from build123d import *

# Parameters (mm, degrees)
SKETCH1_W                 = 8.94
SKETCH1_H                 = 8.96
EXTRUDE1_DEPTH            = 2.85
M5X0_8_TAPPED_HOLE1_D     = 4.2
M5X0_8_TAPPED_HOLE1_DEPTH = 12.4
M5X0_8_TAPPED_HOLE1_TIP   = 1.2618073
CHAMFER1_SIZE             = 1


with BuildPart() as part:
    # Sketch1 → Extrude1 (new body)
    with BuildSketch(Plane(origin=(0, 0, 0), x_dir=(1, 0, 0), z_dir=(0, 1, 0))):
        with Locations((0, -0.02)):
            Rectangle(SKETCH1_W, SKETCH1_H)
    extrude(amount=EXTRUDE1_DEPTH)

    # M5x0.8 Tapped Hole1
    with Locations(Plane(origin=(0, 2.85, 0), x_dir=(1, 0, 0), z_dir=(0, 1, 0))):
        with Locations((0, 0)):
            Hole(M5X0_8_TAPPED_HOLE1_D / 2, depth=M5X0_8_TAPPED_HOLE1_DEPTH)
            with Locations((0, 0, -(M5X0_8_TAPPED_HOLE1_DEPTH + M5X0_8_TAPPED_HOLE1_TIP / 2))):  # 118° drill point
                Cone(0, M5X0_8_TAPPED_HOLE1_D / 2, M5X0_8_TAPPED_HOLE1_TIP, mode=Mode.SUBTRACT)

    # Chamfer1
    chamfer1_edges = [part.edges().sort_by_distance(p)[0] for p in [
        (4.47, 2.85, 0.02),
        (-4.47, 2.85, 0.02),
    ]]
    chamfer(chamfer1_edges, length=CHAMFER1_SIZE)


solid = part.part
Input: part model. Units: mm. Frame: model coordinates. Give positions to 0.01 mm unless a question says otherwise; leave off trailing zeros. Order: outer loops, then holes, each group sorted by start corner. A loop starts at its lowest first (then second) coordinate and runs counter-clockwise, first axis right, second up. Notation, with made-up numbers: (66, 17) -> (88, 17) arc R9 ccw to (88, 29) -> close; hole circle Ø1 at (81, 79). An arc over 180 degrees is marked (long way). Use one line per item in the form item = value.
1) Section C-C, the plane y = 2.1. Return loops of the section in (x, z), and give its area (3 significant figures).
Response values:
outline = (-4.22, -4.46) -> (4.22, -4.46) -> (4.22, 4.5) -> (-4.22, 4.5) -> close; hole circle Ø4.2 at (0, 0)
area = 61.8 mm^2
2) Mould query, pull axis Z, two halves, no side actions, for faces 1 (the cylindrical face through (-2.003, 1.405, -0.631)), 2 (the flat face through (0, 1, 4.5)), 3 (the flat face through (-4.47, 1, 0)). Classes: pulls with the +Z half, pulls with the -Z half, needs draft (parallel to the pull), parting line crosses it, or undercut.
Response values:
face_1 = undercut
face_2 = pulls with the +Z half
face_3 = needs draft
3) Section A-A, the plane z = 0. Return loops of the section in (x, y), and give its area (3 significant figures).
Response values:
outline = (-4.47, 0) -> (-2.1, 0) -> (-2.1, 2.85) -> (-3.47, 2.85) -> (-4.47, 1.85) -> close; (2.1, 0) -> (4.47, 0) -> (4.47, 1.85) -> (3.47, 2.85) -> (2.1, 2.85) -> close
area = 12.5 mm^2
4) Line query: probe 1 along Z at (x, y) = (0, 0.85); probe 2 along X at (y, z) = (1.95, -0.75); probe 3 along Z at (x, y) = (-1, 1.65). Output: solid intervals per line, ascending.
Response values:
probe_1 = -4.46 to -2.1, 2.1 to 4.5
probe_2 = -4.37 to -1.96, 1.96 to 4.37
probe_3 = -4.46 to -1.85, 1.85 to 4.5
5) Section D-D, the plane z = -4. Return loops of the section in (x, y).
Response values:
outline = (-4.47, 0) -> (4.47, 0) -> (4.47, 1.85) -> (3.47, 2.85) -> (-3.47, 2.85) -> (-4.47, 1.85) -> close
6) Section B-B, the plane x = 0. Return loops of the section in (y, z), and give its area (3 significant figures).
Response values:
outline = (0, -4.46) -> (2.85, -4.46) -> (2.85, -2.1) -> (0, -2.1) -> close; (0, 2.1) -> (2.85, 2.1) -> (2.85, 4.5) -> (0, 4.5) -> close
area = 13.6 mm^2
